Can you work these out from the model? Positions are in its coordinate system, mm. Round coordinates to 2 decimals unless told otherwise and drop trailing zeros. Order: outer loops, then holes, each group sorted by start corner. A loop starts at its lowest first (then second) coordinate and runs counter-clockwise, first axis right, second up. Notation, with made-up numbers: (0, 59.25) -> (6, 59.25) arc R27 ccw to (6, 77.25) -> close; hole circle Ø7 at (-34.5, 49.5). An arc over 180 degrees is marked (long way). Use a Markdown table: item, result. Add a question column.
Q1. If we section it at B-B on x = -40: List the corners of the cut face in (y, z) for me, plus the area to 3 significant figures.
Q2. I need wall thicknesses on line 1 along X through (y, z) = (29.5, 0.65); line 2 along X through (y, z) = (29, 1.7); line 3 along Y through (x, z) = (-28.5, 3.7). Which ranges of each line are inside material? Lowest first, please. Write a range as [from, to].
Q3. If we section it at C-C on x = 41.5: List the corners of the cut face in (y, z) for me.
Q4. If we section it at A-A on y = 32: Give the number of separate pieces and of enclosed holes in the cut face, plus the area to 3 significant figures.
```python
from build123d import *

# Parameters (mm, degrees)
EXTRUDE_DEPTH      = 6
EXTRUDE_DEPTH_BACK = 1
CYLINDER_R         = 50
CYLINDER_DEPTH     = 5


with BuildPart() as extrude_body:
    # Sketch → Extrude (new body, two sides)
    with BuildSketch(Plane.XY) as extrude_sk:
        with BuildLine():
            add(Edge.make_bspline(
                [(0, 20.3714), (-19.252262, 51.958269), (-66.21259, 25.005477), (-0.43936, -37.8768)],
                knots=[0, 0, 0, 0, 1, 1, 1, 1], degree=3))
            add(Edge.make_bspline(
                [(0, 20.3714), (19.252262, 51.958269), (66.21259, 25.005477), (-0.43936, -37.8768)],
                knots=[0, 0, 0, 0, 1, 1, 1, 1], degree=3))
        make_face()
    extrude(amount=EXTRUDE_DEPTH)
    extrude(extrude_sk.sketch, amount=-EXTRUDE_DEPTH_BACK)


with BuildPart() as cut:
    # Cylinder → Cylinder (new body)
    with BuildSketch(Plane.XY):
        Circle(CYLINDER_R)
    extrude(amount=CYLINDER_DEPTH)

    # Cut: cut Extrude body
    add(extrude_body.part, mode=Mode.SUBTRACT)


solid = cut.part
```
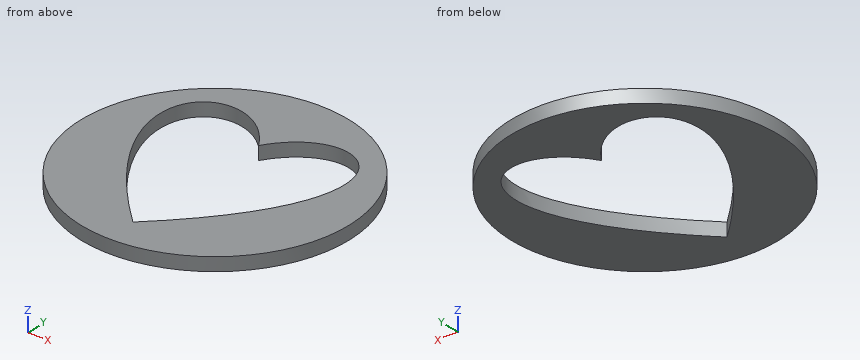
Answer below:
| question | item | result |
|---|---|---|
| 1 | outline | (-30, 0) -> (30, 0) -> (30, 5) -> (-30, 5) -> close |
| 1 | area | 300 mm² |
| 2 | line 1 | [-40.37, -30.04], [-8.22, 8.22], [29.96, 40.37] |
| 2 | line 2 | [-40.73, -30.49], [-7.55, 7.55], [30.4, 40.73] |
| 2 | line 3 | [-41.08, -2.77], [30.88, 41.08] |
| 3 | outline | (-27.89, 0) -> (27.89, 0) -> (27.89, 5) -> (-27.89, 5) -> close |
| 4 | separate pieces | 3 |
| 4 | enclosed holes | 0 |
| 4 | area | 242 mm² |
